from build123d import *

# Parameters (mm, degrees)
BOSS_EXTRUDE1_DEPTH = 304.8
SKETCH2_W           = 25.542619615
SKETCH2_H           = 6.35
CUT_EXTRUDE1_DEPTH  = 6.35
LPATTERN1_COUNT     = 6
LPATTERN1_PITCH     = 50.8
BOSS_EXTRUDE2_DEPTH = 6.35
CUT_EXTRUDE2_DEPTH  = 315.265122799
SKETCH5_R           = 2.0955
CUT_EXTRUDE3_DEPTH  = 315.265122799
CUT_EXTRUDE4_DEPTH  = 315.265122799


with BuildPart() as part:
    # Sketch1 → Boss-Extrude1 (new body)
    with BuildSketch(Plane.XY):
        Polygon((69.147972132, 48.095032857), (110.457150289, 6.7858547), (114.94727835, 11.275982761), (73.638100193, 52.585160918), align=None)
    extrude(amount=BOSS_EXTRUDE1_DEPTH)

    # Sketch2 → Cut-Extrude1 (cut)
    with BuildSketch(Plane(origin=(63.111630555, 63.111630555, 0), x_dir=(0, 0, -1), z_dir=(0.7071067811865472, 0.7071067811865478, 0))):
        with Locations((-266.628690193, -18.061676125)):
            Rectangle(SKETCH2_W, SKETCH2_H)
        with Locations((-266.628690193, -70.131676125)):
            Rectangle(SKETCH2_W, SKETCH2_H)
    cut_extrude1 = extrude(amount=-CUT_EXTRUDE1_DEPTH, mode=Mode.SUBTRACT)

    # LPattern1: Cut-Extrude1 ×6
    with Locations(*[(0, 0, -i * LPATTERN1_PITCH) for i in range(1, LPATTERN1_COUNT)]):
        add(cut_extrude1, mode=Mode.SUBTRACT)

    # Sketch3 → Boss-Extrude2 (add)
    with BuildSketch(Plane(origin=(0, 0, 0), x_dir=(-1, 0, 0), z_dir=(0, 0, -1))):
        Polygon((-84.426151589, 32.816853401), (-93.40640771, 23.83659728), (-97.89653577, 28.32672534), (-88.916279649, 37.306981461), align=None)
    extrude(amount=BOSS_EXTRUDE2_DEPTH)

    # Sketch4 → Cut-Extrude2 (cut, through all)
    with BuildSketch(Plane(origin=(58.621502495, 58.621502495, 0), x_dir=(-0.7071067811865478, 0.7071067811865472, 0), z_dir=(-0.7071067811865472, -0.7071067811865478, 0))):
        Polygon((-55.941380423, 0), (-60.208580423, 0), (-60.208580423, -8.763), (-62.519980423, -8.763), (-62.519980423, -11.938), (-60.208580423, -11.938), (-60.208580423, -15.24), (-55.941380423, -15.24), (-55.941380423, -11.938), (-53.629980423, -11.938), (-53.629980423, -8.763), (-55.941380423, -8.763), align=None)
        Polygon((-26.731380423, 0), (-30.998580423, 0), (-30.998580423, -8.763), (-33.309980423, -8.763), (-33.309980423, -11.938), (-30.998580423, -11.938), (-30.998580423, -15.24), (-26.731380423, -15.24), (-26.731380423, -11.938), (-24.419980423, -11.938), (-24.419980423, -8.763), (-26.731380423, -8.763), align=None)
    extrude(amount=-CUT_EXTRUDE2_DEPTH, mode=Mode.SUBTRACT)

    # Sketch5 → Cut-Extrude3 (cut, through all)
    with BuildSketch(Plane(origin=(58.621502495, 58.621502495, 0), x_dir=(-0.7071067811865478, 0.7071067811865472, 0), z_dir=(-0.7071067811865472, -0.7071067811865478, 0))):
        with Locations(Location((-18.061676125, -38.1, 0), (0, 0, 180))):
            Circle(SKETCH5_R)
        with Locations(Location((-18.061676125, -292.1, 0), (0, 0, 180))):
            Circle(SKETCH5_R)
    cut_extrude3 = extrude(amount=-CUT_EXTRUDE3_DEPTH, mode=Mode.SUBTRACT)

    # Mirror1: Cut-Extrude3 across plane
    add(cut_extrude3.mirror(Plane(origin=(31.181058716, -31.181058716, 0), x_dir=(0, 0, 1), z_dir=(0.7071067811865478, -0.7071067811865472, 0))), mode=Mode.SUBTRACT)

    # Sketch6 → Cut-Extrude4 (cut, through all)
    with BuildSketch(Plane(origin=(58.621502495, 58.621502495, 0), x_dir=(-0.7071067811865478, 0.7071067811865472, 0), z_dir=(-0.7071067811865472, -0.7071067811865478, 0))):
        Polygon((-21.236676125, -65.562290193), (-21.236676125, -61.295090193), (-29.999676125, -61.295090193), (-29.999676125, -58.983690193), (-33.174676125, -58.983690193), (-33.174676125, -61.295090193), (-36.476676125, -61.295090193), (-36.476676125, -65.562290193), (-33.174676125, -65.562290193), (-33.174676125, -67.873690193), (-29.999676125, -67.873690193), (-29.999676125, -65.562290193), align=None)
        Polygon((-21.236676125, -217.962290193), (-21.236676125, -213.695090193), (-29.999676125, -213.695090193), (-29.999676125, -211.383690193), (-33.174676125, -211.383690193), (-33.174676125, -213.695090193), (-36.476676125, -213.695090193), (-36.476676125, -217.962290193), (-33.174676125, -217.962290193), (-33.174676125, -220.273690193), (-29.999676125, -220.273690193), (-29.999676125, -217.962290193), align=None)
    cut_extrude4 = extrude(amount=-CUT_EXTRUDE4_DEPTH, mode=Mode.SUBTRACT)

    # Mirror2: Cut-Extrude4 across plane
    add(cut_extrude4.mirror(Plane(origin=(31.181058716, -31.181058716, 0), x_dir=(0, 0, 1), z_dir=(0.7071067811865478, -0.7071067811865472, 0))), mode=Mode.SUBTRACT)


solid = part.part
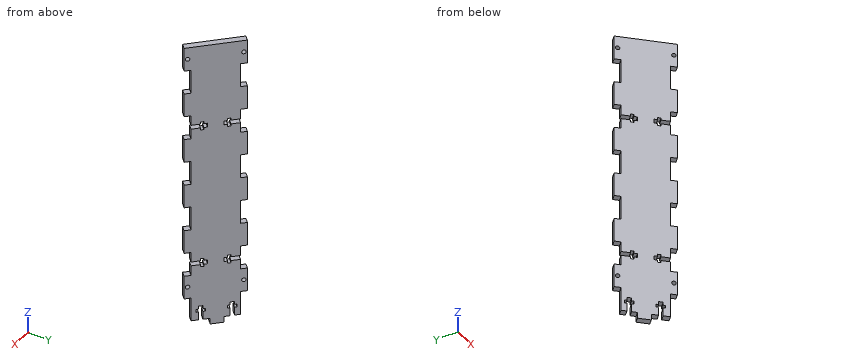
Build history of the part. All positions in model axes, mm. Give positions to 0.01 mm unless a question says otherwise; leave off trailing zeros. Order: outer loops, then holes, each group sorted by start corner. A loop starts at its lowest first (then second) coordinate and runs counter-clockwise, first axis right, second up. Notation, with made-up numbers: M 48.25,-5 L 86.25,-5 A18 ccw 86.25,14 Z; hole C -13,64 d11. An arc over 180 degrees is marked long. Put each result on its own line as item: value.
Item 1: Slice it at A-A, the plane z = 200. Write the cut outline in (x, y), plus the area to 3 significant figures.
From the geometry:
outline: M 69.15,48.1 L 110.46,6.79 L 114.95,11.28 L 73.64,52.59 Z
area: 371 mm2
Item 2: Slice it at B-B, the plane z = 73. Write the cut outline in (x, y), plus the area to 3 significant figures.
From the geometry:
outline: M 73.64,43.6 L 105.97,11.28 L 110.46,15.77 L 78.13,48.1 Z
area: 290 mm2
Item 3: Flat gauge pins, fed straight in: pin 1 Ø1.5 at (x, z) = (100.5, 57) entering from +Y; pin 2 Ø4.5 at (x, y) = (110, 13.5) entering from -Z; pin 3 Ø1.5 at (x, z) = (76.5, 162) entering from -Y. Where does each tip first touch, or does it go through?
From the geometry:
pin 1: stops at y = 26.47
pin 2: stops at z = 0
pin 3: stops at y = 39.99
Item 4: Probe line 1 (Z direction, x = 80, y = 41); line 2 (Y direction, x = 110.5, z = 200.5); line 3 (Y direction, x = 74, z = 38.5). List the from-to ranges inside material, lowest first. Write a range as [from, to].
From the geometry:
line 1: z = [15.24, 61.3], [65.56, 213.7], [217.96, 304.8]
line 2: y = [6.83, 15.72]
line 3: y = [43.24, 45.55], [51.37, 52.22]
